from build123d import *

# Parameters (mm, degrees)
SKETCH_1_W          = 32
SKETCH_1_H          = 18
SKETCH_1_R          = 1.2
SKETCH_1_W_2        = 23
SKETCH_1_H_2        = 12
EXTRUDE_1_DEPTH     = 3
CUT_EXTRUDE_1_REACH = 20.601
SKETCH_2_R          = 1
SKETCH_4_W          = 32
SKETCH_4_H          = 15
SKETCH_4_R          = 1.45
EXTRUDE_2_DEPTH     = 3
FILLET_1_R          = 2


with BuildPart() as part:
    # 草图1 → 凸台-拉伸1 (new body)
    with BuildSketch(Plane(origin=(0, 0, 0), x_dir=(1, 0, 0), z_dir=(0, 1, 0))):
        Rectangle(SKETCH_1_W, SKETCH_1_H)
        with Locations(Location((-14, 3.5, 0), (0, 0, 270))):
            Circle(SKETCH_1_R, mode=Mode.SUBTRACT)
        with Locations(Location((-14, -3.5, 0), (0, 0, 270))):
            Circle(SKETCH_1_R, mode=Mode.SUBTRACT)
        with Locations(Location((14, 3.5, 0), (0, 0, 270))):
            Circle(SKETCH_1_R, mode=Mode.SUBTRACT)
        with Locations(Location((14, -3.5, 0), (0, 0, 270))):
            Circle(SKETCH_1_R, mode=Mode.SUBTRACT)
        Rectangle(SKETCH_1_W_2, SKETCH_1_H_2, mode=Mode.SUBTRACT)
    extrude(amount=EXTRUDE_1_DEPTH)

    # 草图2 → 切除-拉伸1 (cut, up to next)
    with BuildSketch(Plane(origin=(0, 3, 0), x_dir=(1, 0, 0), z_dir=(0, 1, 0)), mode=Mode.PRIVATE) as cut_extrude_1_sk1:
        with Locations((-11.5, 6)):
            Circle(SKETCH_2_R)
    cut_extrude_1_tool1 = extrude(cut_extrude_1_sk1.sketch, amount=-CUT_EXTRUDE_1_REACH, mode=Mode.PRIVATE) & part.part
    # 草图2 → 切除-拉伸1 (cut, up to next)
    with BuildSketch(Plane(origin=(0, 3, 0), x_dir=(1, 0, 0), z_dir=(0, 1, 0)), mode=Mode.PRIVATE) as cut_extrude_1_sk2:
        with Locations((-11.5, -6)):
            Circle(SKETCH_2_R)
    cut_extrude_1_tool2 = extrude(cut_extrude_1_sk2.sketch, amount=-CUT_EXTRUDE_1_REACH, mode=Mode.PRIVATE) & part.part
    # 草图2 → 切除-拉伸1 (cut, up to next)
    with BuildSketch(Plane(origin=(0, 3, 0), x_dir=(1, 0, 0), z_dir=(0, 1, 0)), mode=Mode.PRIVATE) as cut_extrude_1_sk3:
        with Locations((11.5, -6)):
            Circle(SKETCH_2_R)
    cut_extrude_1_tool3 = extrude(cut_extrude_1_sk3.sketch, amount=-CUT_EXTRUDE_1_REACH, mode=Mode.PRIVATE) & part.part
    # 草图2 → 切除-拉伸1 (cut, up to next)
    with BuildSketch(Plane(origin=(0, 3, 0), x_dir=(1, 0, 0), z_dir=(0, 1, 0)), mode=Mode.PRIVATE) as cut_extrude_1_sk4:
        with Locations((11.5, 6)):
            Circle(SKETCH_2_R)
    cut_extrude_1_tool4 = extrude(cut_extrude_1_sk4.sketch, amount=-CUT_EXTRUDE_1_REACH, mode=Mode.PRIVATE) & part.part
    add(cut_extrude_1_tool1.solids().sort_by_distance((-11.5, 3, -6))[0], mode=Mode.SUBTRACT)
    add(cut_extrude_1_tool2.solids().sort_by_distance((-11.5, 3, 6))[0], mode=Mode.SUBTRACT)
    add(cut_extrude_1_tool3.solids().sort_by_distance((11.5, 3, 6))[0], mode=Mode.SUBTRACT)
    add(cut_extrude_1_tool4.solids().sort_by_distance((11.5, 3, -6))[0], mode=Mode.SUBTRACT)

    # 草图4 → 凸台-拉伸2 (add)
    with BuildSketch(Plane(origin=(0, 3, 0), x_dir=(1, 0, 0), z_dir=(0, 1, 0))):
        with Locations((0, -16.5)):
            Rectangle(SKETCH_4_W, SKETCH_4_H)
        with Locations(Location((-11, -16.5, 0), (0, 0, 270))):
            Circle(SKETCH_4_R, mode=Mode.SUBTRACT)
        with Locations(Location((11, -16.5, 0), (0, 0, 270))):
            Circle(SKETCH_4_R, mode=Mode.SUBTRACT)
    extrude(amount=-EXTRUDE_2_DEPTH)

    # 圆角1
    fillet_1_edges = [part.edges().sort_by_distance(p)[0] for p in [
        (-16, 1.5, -9),
        (16, 1.5, -9),
        (-16, 1.5, 24),
        (16, 1.5, 24),
    ]]
    fillet(fillet_1_edges, radius=FILLET_1_R)


solid = part.part
Source: CAD feature listing. Evaluate the final solid. Frame: model axes, mm. A direction names the side the tool comes from. Coordinates: 2 decimals unless noted, no trailing zeros. Write each loop counter-clockwise with the first axis right and the second up, starting at its lowest first coordinate (ties: lowest second). Pieces come first, ordered by that corner, then holes. Notation, with made-up numbers: M 11,-36 L 67,-36 A25 cw 67,-8 Z; hole C 34,-25 d9. An arc over 180 degrees is marked long. Use a Markdown table: item, result.
1) Section A-A, the plane z = -1. Output: boundary loops of the cut face in (x, y).
Conclusion:
| item | result |
|---|---|
| outline | M -16,0 L -11.5,0 L -11.5,3 L -16,3 Z; M 11.5,0 L 16,0 L 16,3 L 11.5,3 Z |
2) First-contact query: pin 1 Ø1.8 at (x, z) = (-11.5, -6) entering from -Y. Flat tip, straight axial feed; report the tip coordinate or a pass-through.
Conclusion:
| item | result |
|---|---|
| pin 1 | passes through |
3) Reachability of faces 1 (the cylindrical face through (15.43, 1.48, 23.4)), 2 (the flat face through (-11.5, 1, 0)) from +Z, -Z, +X, -X, +Y, -Y: full face, straight path, thin tool, end or side. Return the list, or none.
Conclusion:
| item | result |
|---|---|
| face 1 | +Z, +X, +Y, -Y |
| face 2 | +Y, -Y |
4) Section B-B, the plane x = 3. Output: boundary loops of the cut face in (y, z), then the cut area to 3 significant figures.
Conclusion:
| item | result |
|---|---|
| outline | M 0,-9 L 3,-9 L 3,-6 L 0,-6 Z; M 0,6 L 3,6 L 3,24 L 0,24 Z |
| area | 63.0 mm^2 |
5) Mould query, pull axis Z, two halves, no side actions, for faces 3 (the flat face through (0, 2, 24)), 4 (the cylindrical face through (-12.23, 1.521, 6.683)), 5 (the flat face through (0, 1, -9)). Classes: pulls with the +Z half, pulls with the -Z half, needs draft (parallel to the pull), parting line crosses it, or undercut.
Conclusion:
| item | result |
|---|---|
| face 3 | pulls with the +Z half |
| face 4 | undercut |
| face 5 | pulls with the -Z half |
6) Section D-D, the plane z = 15.5. Output: boundary loops of the cut face in (x, y).
Conclusion:
| item | result |
|---|---|
| outline | M -16,0 L -12.05,0 L -12.05,3 L -16,3 Z; M -9.95,0 L 9.95,0 L 9.95,3 L -9.95,3 Z; M 12.05,0 L 16,0 L 16,3 L 12.05,3 Z |
7) Ray query, L1, parallel to X at y = 1.5, z = 3.5; L2, parallel to X at y = 1.05, z = 16.5; L3, parallel to Z at x = 8.5, y = 1. Return the intervals inside material, ascending.
Conclusion:
| item | result |
|---|---|
| L1 | x = -16 to -15.2, -12.8 to -11.5, 11.5 to 12.8, 15.2 to 16 |
| L2 | x = -16 to -12.45, -9.55 to 9.55, 12.45 to 16 |
| L3 | z = -9 to -6, 6 to 24 |
8) Section C-C, the plane y = 0.85. Output: boundary loops of the cut face in (x, z), then the cut area to 3 significant figures.
Conclusion:
| item | result |
|---|---|
| outline | M -16,-7 A2 ccw -14,-9 L 14,-9 A2 ccw 16,-7 L 16,22 A2 ccw 14,24 L -14,24 A2 ccw -16,22 Z; hole C -14,-3.5 d2.4; hole C -14,3.5 d2.4; hole C -11,16.5 d2.9; hole M -11.5,-5 A1 ccw long -10.5,-6 L 10.5,-6 A1 ccw long 11.5,-5 L 11.5,5 A1 ccw long 10.5,6 L -10.5,6 A1 ccw long -11.5,5 Z; hole C 11,16.5 d2.9; hole C 14,-3.5 d2.4; hole C 14,3.5 d2.4 |
| area | 736 mm^2 |
